CAD build for the part. Positions are in the model's coordinates, mm. A direction names the side the tool comes from. Give positions to 0.01 mm unless a question says otherwise; leave off trailing zeros. Write each loop counter-clockwise with the first axis right and the second up, starting at its lowest first coordinate (ties: lowest second). Pieces come first, ordered by that corner, then holes. Notation, with made-up numbers: (30, -3.75) - (88, -3.75) arc R32 ccw to (88, 33.25) - close; hole circle Ø3 at (66, 88). An arc over 180 degrees is marked (long way). Answer as a JSON object with one key per item and string values.
from build123d import *

# Parameters (mm, degrees)
CROQUIS1_R              = 5.3
SALIENTE_EXTRUIR1_DEPTH = 2
CROQUIS2_R              = 1.8
CORTAR_EXTRUIR1_DEPTH   = 2
CROQUIS3_W              = 24.61
CROQUIS3_H              = 60
SALIENTE_EXTRUIR2_DEPTH = 2
CROQUIS4_R              = 5.3
CROQUIS4_R_2            = 1.8
SALIENTE_EXTRUIR3_DEPTH = 2
CORTAR_EXTRUIR2_REACH   = 48.282
CROQUIS5_R              = 5.4
CROQUIS5_R_2            = 1.8
CROQUIS6_W              = 24.61
CROQUIS6_H              = 60
SALIENTE_EXTRUIR4_DEPTH = 1
CORTAR_EXTRUIR3_REACH   = 49.282
CROQUIS7_R              = 5.4
CROQUIS7_R_2            = 1.8
REDONDEO1_R             = 2


with BuildPart() as part:
    # Croquis1 → Saliente-Extruir1 (new body)
    with BuildSketch(Plane(origin=(0, 0, 0), x_dir=(1, 0, 0), z_dir=(0, 1, 0))):
        with BuildLine():
            Line((-10.994972408, -15.789813385), (14.087680331, -13.105147381))
            ThreePointArc((14.087680331, -13.105147381), (25.196689721, 4.143672323), (5.987949996, 11.351736486))
            Line((5.987949996, 11.351736486), (-10.55372573, 9.581234979))
            Line((-10.55372573, 9.581234979), (-26.287258722, -9.342507769))
            Line((-26.287258722, -9.342507769), (-22.837316291, -12.210850664))
            ThreePointArc((-22.837316291, -12.210850664), (-17.278998917, -15.200972796), (-10.994972408, -15.789813385))
        make_face()
        with Locations((12.685, 0)):
            Circle(CROQUIS1_R, mode=Mode.SUBTRACT)
    extrude(amount=SALIENTE_EXTRUIR1_DEPTH)

    # Croquis2 → Cortar-Extruir1 (cut)
    with BuildSketch(Plane(origin=(0, 2, 0), x_dir=(1, 0, 0), z_dir=(0, 1, 0))):
        with Locations((6.092709789, -8.172619517)):
            Circle(CROQUIS2_R)
        with Locations((20.857619517, -6.592290211)):
            Circle(CROQUIS2_R)
        with Locations((19.277290211, 8.172619517)):
            Circle(CROQUIS2_R)
        with Locations((4.512380483, 6.592290211)):
            Circle(CROQUIS2_R)
    extrude(amount=-CORTAR_EXTRUIR1_DEPTH, mode=Mode.SUBTRACT)

    # Croquis3 → Saliente-Extruir2 (add)
    with BuildSketch(Plane(origin=(-10.950288723, 0, -9.104262893), x_dir=(-0.639314628, 0, 0.768945256), z_dir=(-0.768945256, 0, -0.639314628))):
        with Locations((11.684706055, 30)):
            Rectangle(CROQUIS3_W, CROQUIS3_H)
    extrude(amount=SALIENTE_EXTRUIR2_DEPTH)

    # Croquis4 → Saliente-Extruir3 (add)
    with BuildSketch(Plane(origin=(0, 60, 0), x_dir=(1, 0, 0), z_dir=(0, 1, 0))):
        with BuildLine():
            Line((14.087680331, -13.105147381), (-10.994972408, -15.789813385))
            ThreePointArc((-10.994972408, -15.789813385), (-17.278998917, -15.200972796), (-22.837316291, -12.210850664))
            Line((-22.837316291, -12.210850664), (-26.287258722, -9.342507769))
            Line((-26.287258722, -9.342507769), (-10.55372573, 9.581234979))
            Line((-10.55372573, 9.581234979), (5.987949996, 11.351736486))
            ThreePointArc((5.987949996, 11.351736486), (25.196689721, 4.143672323), (14.087680331, -13.105147381))
        make_face()
        with Locations((12.685, 0)):
            Circle(CROQUIS4_R, mode=Mode.SUBTRACT)
        with Locations((4.512380483, 6.592290211)):
            Circle(CROQUIS4_R_2, mode=Mode.SUBTRACT)
        with Locations((19.277290211, 8.172619517)):
            Circle(CROQUIS4_R_2, mode=Mode.SUBTRACT)
        with Locations((20.857619517, -6.592290211)):
            Circle(CROQUIS4_R_2, mode=Mode.SUBTRACT)
        with Locations((6.092709789, -8.172619517)):
            Circle(CROQUIS4_R_2, mode=Mode.SUBTRACT)
    extrude(amount=-SALIENTE_EXTRUIR3_DEPTH)

    # Croquis5 → Cortar-Extruir2 (cut, up to next)
    with BuildSketch(Plane(origin=(-12.488179234, 0, -10.382892148), x_dir=(-0.639314628, 0, 0.768945256), z_dir=(-0.768945256, 0, -0.639314628)), mode=Mode.PRIVATE) as cortar_extruir2_sk1:
        with Locations((11.684706055, 30)):
            Circle(CROQUIS5_R)
    cortar_extruir2_tool1 = extrude(cortar_extruir2_sk1.sketch, amount=-CORTAR_EXTRUIR2_REACH, mode=Mode.PRIVATE) & part.part
    add(cortar_extruir2_tool1.solids().sort_by_distance((-19.958383, 30, -1.397993))[0], mode=Mode.SUBTRACT)
    # Croquis5 → Cortar-Extruir2 (cut, up to next)
    with BuildSketch(Plane(origin=(-12.488179234, 0, -10.382892148), x_dir=(-0.639314628, 0, 0.768945256), z_dir=(-0.768945256, 0, -0.639314628)), mode=Mode.PRIVATE) as cortar_extruir2_sk2:
        with Locations((19.109327257, 37.424621202)):
            Circle(CROQUIS5_R_2)
    cortar_extruir2_tool2 = extrude(cortar_extruir2_sk2.sketch, amount=-CORTAR_EXTRUIR2_REACH, mode=Mode.PRIVATE) & part.part
    add(cortar_extruir2_tool2.solids().sort_by_distance((-24.705052, 37.424621, 4.311134))[0], mode=Mode.SUBTRACT)
    # Croquis5 → Cortar-Extruir2 (cut, up to next)
    with BuildSketch(Plane(origin=(-12.488179234, 0, -10.382892148), x_dir=(-0.639314628, 0, 0.768945256), z_dir=(-0.768945256, 0, -0.639314628)), mode=Mode.PRIVATE) as cortar_extruir2_sk3:
        with Locations((19.109327257, 22.575378798)):
            Circle(CROQUIS5_R_2)
    cortar_extruir2_tool3 = extrude(cortar_extruir2_sk3.sketch, amount=-CORTAR_EXTRUIR2_REACH, mode=Mode.PRIVATE) & part.part
    add(cortar_extruir2_tool3.solids().sort_by_distance((-24.705052, 22.575379, 4.311134))[0], mode=Mode.SUBTRACT)
    # Croquis5 → Cortar-Extruir2 (cut, up to next)
    with BuildSketch(Plane(origin=(-12.488179234, 0, -10.382892148), x_dir=(-0.639314628, 0, 0.768945256), z_dir=(-0.768945256, 0, -0.639314628)), mode=Mode.PRIVATE) as cortar_extruir2_sk4:
        with Locations((4.260084852, 22.575378798)):
            Circle(CROQUIS5_R_2)
    cortar_extruir2_tool4 = extrude(cortar_extruir2_sk4.sketch, amount=-CORTAR_EXTRUIR2_REACH, mode=Mode.PRIVATE) & part.part
    add(cortar_extruir2_tool4.solids().sort_by_distance((-15.211714, 22.575379, -7.10712))[0], mode=Mode.SUBTRACT)
    # Croquis5 → Cortar-Extruir2 (cut, up to next)
    with BuildSketch(Plane(origin=(-12.488179234, 0, -10.382892148), x_dir=(-0.639314628, 0, 0.768945256), z_dir=(-0.768945256, 0, -0.639314628)), mode=Mode.PRIVATE) as cortar_extruir2_sk5:
        with Locations((4.260084852, 37.424621202)):
            Circle(CROQUIS5_R_2)
    cortar_extruir2_tool5 = extrude(cortar_extruir2_sk5.sketch, amount=-CORTAR_EXTRUIR2_REACH, mode=Mode.PRIVATE) & part.part
    add(cortar_extruir2_tool5.solids().sort_by_distance((-15.211714, 37.424621, -7.10712))[0], mode=Mode.SUBTRACT)

    # Croquis6 → Saliente-Extruir4 (add)
    with BuildSketch(Plane(origin=(-12.488179234, 0, -10.382892148), x_dir=(0.639314628, 0, -0.768945256), z_dir=(0.768945256, 0, 0.639314628))):
        with Locations((-11.684706055, 30)):
            Rectangle(CROQUIS6_W, CROQUIS6_H)
    extrude(amount=-SALIENTE_EXTRUIR4_DEPTH)

    # Croquis7 → Cortar-Extruir3 (cut, up to next)
    with BuildSketch(Plane(origin=(-13.25712449, 0, -11.022206776), x_dir=(-0.639314628, 0, 0.768945256), z_dir=(-0.768945256, 0, -0.639314628)), mode=Mode.PRIVATE) as cortar_extruir3_sk1:
        with Locations((11.684706055, 30)):
            Circle(CROQUIS7_R)
    cortar_extruir3_tool1 = extrude(cortar_extruir3_sk1.sketch, amount=-CORTAR_EXTRUIR3_REACH, mode=Mode.PRIVATE) & part.part
    add(cortar_extruir3_tool1.solids().sort_by_distance((-20.727328, 30, -2.037307))[0], mode=Mode.SUBTRACT)
    # Croquis7 → Cortar-Extruir3 (cut, up to next)
    with BuildSketch(Plane(origin=(-13.25712449, 0, -11.022206776), x_dir=(-0.639314628, 0, 0.768945256), z_dir=(-0.768945256, 0, -0.639314628)), mode=Mode.PRIVATE) as cortar_extruir3_sk2:
        with Locations((4.260084852, 37.424621202)):
            Circle(CROQUIS7_R_2)
    cortar_extruir3_tool2 = extrude(cortar_extruir3_sk2.sketch, amount=-CORTAR_EXTRUIR3_REACH, mode=Mode.PRIVATE) & part.part
    add(cortar_extruir3_tool2.solids().sort_by_distance((-15.980659, 37.424621, -7.746435))[0], mode=Mode.SUBTRACT)
    # Croquis7 → Cortar-Extruir3 (cut, up to next)
    with BuildSketch(Plane(origin=(-13.25712449, 0, -11.022206776), x_dir=(-0.639314628, 0, 0.768945256), z_dir=(-0.768945256, 0, -0.639314628)), mode=Mode.PRIVATE) as cortar_extruir3_sk3:
        with Locations((19.109327257, 37.424621202)):
            Circle(CROQUIS7_R_2)
    cortar_extruir3_tool3 = extrude(cortar_extruir3_sk3.sketch, amount=-CORTAR_EXTRUIR3_REACH, mode=Mode.PRIVATE) & part.part
    add(cortar_extruir3_tool3.solids().sort_by_distance((-25.473997, 37.424621, 3.67182))[0], mode=Mode.SUBTRACT)
    # Croquis7 → Cortar-Extruir3 (cut, up to next)
    with BuildSketch(Plane(origin=(-13.25712449, 0, -11.022206776), x_dir=(-0.639314628, 0, 0.768945256), z_dir=(-0.768945256, 0, -0.639314628)), mode=Mode.PRIVATE) as cortar_extruir3_sk4:
        with Locations((19.109327257, 22.575378798)):
            Circle(CROQUIS7_R_2)
    cortar_extruir3_tool4 = extrude(cortar_extruir3_sk4.sketch, amount=-CORTAR_EXTRUIR3_REACH, mode=Mode.PRIVATE) & part.part
    add(cortar_extruir3_tool4.solids().sort_by_distance((-25.473997, 22.575379, 3.67182))[0], mode=Mode.SUBTRACT)
    # Croquis7 → Cortar-Extruir3 (cut, up to next)
    with BuildSketch(Plane(origin=(-13.25712449, 0, -11.022206776), x_dir=(-0.639314628, 0, 0.768945256), z_dir=(-0.768945256, 0, -0.639314628)), mode=Mode.PRIVATE) as cortar_extruir3_sk5:
        with Locations((4.260084852, 22.575378798)):
            Circle(CROQUIS7_R_2)
    cortar_extruir3_tool5 = extrude(cortar_extruir3_sk5.sketch, amount=-CORTAR_EXTRUIR3_REACH, mode=Mode.PRIVATE) & part.part
    add(cortar_extruir3_tool5.solids().sort_by_distance((-15.980659, 22.575379, -7.746435))[0], mode=Mode.SUBTRACT)

    # Redondeo1
    redondeo1_edges = [part.edges().sort_by_distance(p)[0] for p in [
        (-20.727327994, 60, -2.037307489),
        (-18.420492226, 2, -0.119363605),
        (-18.420492226, 58, -0.119363605),
        (-20.727327994, 0, -2.037307489),
    ]]
    fillet(redondeo1_edges, radius=REDONDEO1_R)


solid = part.part
Item 1: Flat gauge pins, fed straight in: P1, Ø1.5, axis at x = -16.5, z = -5.5, coming from the -Y side; P2, Ø1.5, axis at x = -18.5, z = -8, coming from the +Y side (3 decimals); P3, Ø12, axis at y = 42.5, z = 11, coming from the +X side; P4, Ø5, axis at y = 22.5, z = -4, coming from the -X side. Where does each tip first touch, or does it go through?
Entries:
{"P1": "y = 0.01", "P2": "through", "P3": "x = -22.68", "P4": "x = -21.17"}
Item 2: Mould opens along Z. For faces 4 (the flat face through (0, 2, 1)), 5 (the cylindrical face through (19.06, 59.01, 6.51)), 6 (the cylindrical face through (25.296, 0.986, -3.83)), 7 (the flat face through (1.371, 0.986, 14.466)) say: +Z half, -Z half, draft (parallel to the pull), parting line (faces both ways), or undercut.
Entries:
{"face 4": "draft", "face 5": "undercut", "face 6": "parting line", "face 7": "+Z half"}
Item 3: Cut at C-C (z = 0). State how many separate pieces and enclosed holes the cut face has, and give its area (3 significant figures).
Entries:
{"separate pieces": "4", "enclosed holes": "0", "area": "329 mm2"}
Item 4: Which spindle directions (+Z, -Z, +X, -X, +Y, -Y) get a long thin tool onto all of the face, cutting with end or side? Do faces 1 (the cylindrical face through (-17.42, 2.57, -0.38)), 2 (the flat face through (-2.17, 1.08, -10.48)), 3 (the flat face through (-24.334, 30.392, 2.3)). Say none if no direction does.
Entries:
{"face 1": "+Z, +X", "face 2": "-Z, +Y, -Y", "face 3": "-Z, -X, +Y, -Y"}
Item 5: Cut at B-B (x = -7). Give the cut face in (y, z).
Entries:
{"outline": "(0, -9.96) - (2, -9.96) - (2, 15.36) - (0, 15.36) - close; (58, -9.96) - (60, -9.96) - (60, 15.36) - (58, 15.36) - close"}
Item 6: Cut at D-D (y = 41.5). Give the cut face in (x, z), and give its area (3 significant figures).
Entries:
{"outline": "(-28.59, 7.42) - (-12.86, -11.5) - (-10.55, -9.58) - (-26.29, 9.34) - close", "area": "73.8 mm2"}
Item 7: Probe line 1 (Y direction, x = 3, z = -5.25); line 2 (Y direction, x = -17.5, z = -4); line 3 (X direction, y = 0.5, z = 0) (3 decimals). List the from-to ranges inside material, lowest first. Write a range as from..to.
Entries:
{"line 1": "0..2, 58..60", "line 2": "0.16..25.95, 34.05..59.84", "line 3": "-21.541..7.385, 17.985..25.865"}
Item 8: Cut at A-A (y = 26). Give the cut face in (x, z).
Entries:
{"outline": "(-28.59, 7.42) - (-23.05, 0.75) - (-20.74, 2.67) - (-26.29, 9.34) - close; (-18.41, -4.83) - (-12.86, -11.5) - (-10.55, -9.58) - (-16.1, -2.91) - close"}
